For this review, take the finished solid that the model builds, in its own axes (mm). Face numbers are marked on the shaded views. A direction names the side the tool comes from. Give positions to 0.01 mm unless a question says otherwise; leave off trailing zeros. Write each loop counter-clockwise with the first axis right and the second up, starting at its lowest first coordinate (ties: lowest second). Pieces come first, ordered by that corner, then holes.
Q1. We need section D-D (z = -11.5). Write out the cut boundary in (x, y), then the cut area to 3 significant figures.
Q2. We need section B-B (z = 9). Write out the cut boundary in (x, y) (3 decimals), then the cut area to 3 significant figures.
Q3. Insertion check: P1, Ø6, axis at y = 54.5, z = 26, coming from the +X side; P2, Ø6.5, axis at x = 22.5, z = 34, coming from the +Y side; P3, Ø10, axis at y = 54, z = 25.5, coming from the -X side; P4, Ø12, axis at x = 4.5, z = 14.5, coming from the -Y side. Each pin has a flat end and moves straight along its axis. Give the tip position at first contact, or say it passes through.
Q4. Mouldability with a two-part tool opening along Y and no side actions: class the marked faces 1, 2 and 3 as released by +Y, released by -Y, zero draft, split by the parting line, or undercut.
Q5. We need section C-C (y = 0). Write out the cut boundary in (x, z), then the cut area to 3 significant figures.
Q6. We need section A-A (x = 0). Write out the cut boundary in (y, z), then the cut area to 3 significant figures.
Q7. Machinability: for the marked faces 4, 5 and 6, which of the approach directions +Z, -Z, +X, -X, +Y, -Y give a long, thin tool a straight path to every point of the face, cutting with its end or side? Answer none if there is none.
Q8. For line 1 (Z direction, x = 11, y = 32.5); line 2 (Y direction, x = 0, z = 17); line 3 (Z direction, x = 0, y = -19), list the stretches that pass through material, from the lowest coordinate up.
```python
from build123d import *

# Parameters (mm, degrees)
SKETCH1_R           = 30
SKETCH1_R_2         = 17.5
BOSS_EXTRUDE1_DEPTH = 38
BOSS_EXTRUDE2_START = -33
BOSS_EXTRUDE2_DEPTH = 33
SKETCH6_W           = 11
SKETCH6_H           = 36.919601085
BOSS_EXTRUDE3_DEPTH = 41.84
SKETCH8_R           = 5.835
CUT_EXTRUDE2_DEPTH  = 41.84
BOSS_EXTRUDE4_DEPTH = 11
SKETCH13_W          = 14
SKETCH13_H          = 10
BOSS_EXTRUDE7_DEPTH = 55
SKETCH14_W          = 5
SKETCH14_H          = 14
CUT_EXTRUDE3_DEPTH  = 2
BOSS_EXTRUDE8_DEPTH = 10
CUT_EXTRUDE4_DEPTH  = 100.425509369
SKETCH18_W          = 27.083405909
SKETCH18_H          = 15
CUT_EXTRUDE5_DEPTH  = 6


with BuildPart() as part:
    # Sketch1 → Boss-Extrude1 (new body)
    with BuildSketch(Plane.XY):
        Circle(SKETCH1_R)
        Circle(SKETCH1_R_2, mode=Mode.SUBTRACT)
    extrude(amount=BOSS_EXTRUDE1_DEPTH)

    # Sketch3 → Boss-Extrude2 (add)
    with BuildSketch(Plane.XY.offset(38).offset(BOSS_EXTRUDE2_START)):
        with BuildLine():
            Line((5, 29.580398915), (5, 66.5))
            Line((5, 66.5), (-5, 66.5))
            Line((-5, 66.5), (-5, 29.580398915))
            ThreePointArc((-5, 29.580398915), (0, 30), (5, 29.580398915))
        make_face()
    extrude(amount=BOSS_EXTRUDE2_DEPTH)

    # Sketch6 → Boss-Extrude3 (add)
    with BuildSketch(Plane(origin=(5, 0, 0), x_dir=(0, 0, -1), z_dir=(1, 0, 0))):
        with Locations((-10.5, 48.040199458)):
            Rectangle(SKETCH6_W, SKETCH6_H)
    extrude(amount=BOSS_EXTRUDE3_DEPTH)

    # Sketch8 → Cut-Extrude2 (cut)
    with BuildSketch(Plane.XY.offset(16)):
        with BuildLine():
            Line((38.535426242, 49.92600948), (19.843134833, 28.5))
            Line((19.843134833, 28.5), (19.843134833, 22.5))
            Line((19.843134833, 22.5), (50.730835644, 21.613123559))
            Line((50.730835644, 21.613123559), (58.316291642, 73.170252493))
            Line((58.316291642, 73.170252493), (32.080152152, 77.030302224))
            Line((32.080152152, 77.030302224), (31, 66.5))
            ThreePointArc((31, 66.5), (40.103293503, 60.638846144), (38.535426242, 49.92600948))
        make_face()
        with Locations((31, 56.5)):
            Circle(SKETCH8_R)
    extrude(amount=-CUT_EXTRUDE2_DEPTH, mode=Mode.SUBTRACT)

    # Sketch11 → Boss-Extrude4 (add)
    with BuildSketch(Plane(origin=(0, 0, 5), x_dir=(-1, 0, 0), z_dir=(0, 0, -1))):
        with BuildLine():
            Line((-19.843134833, 22.5), (-19.843134833, 28.5))
            Line((-19.843134833, 28.5), (-20.785686986, 29.580398915))
            Line((-20.785686986, 29.580398915), (-5, 29.580398915))
            ThreePointArc((-5, 29.580398915), (-12.91620491, 27.077142588), (-19.843134833, 22.5))
        make_face()
    extrude(amount=-BOSS_EXTRUDE4_DEPTH)

    # Sketch13 → Boss-Extrude7 (add)
    with BuildSketch(Plane.ZY.offset(5)):
        with Locations((12, 34.580398915)):
            Rectangle(SKETCH13_W, SKETCH13_H)
    extrude(amount=BOSS_EXTRUDE7_DEPTH)

    # Sketch14 → Cut-Extrude3 (cut)
    with BuildSketch(Plane(origin=(0, 39.580398915, 0), x_dir=(1, 0, 0), z_dir=(0, 1, 0))):
        with Locations((-7.5, -12)):
            Rectangle(SKETCH14_W, SKETCH14_H)
    extrude(amount=-CUT_EXTRUDE3_DEPTH, mode=Mode.SUBTRACT)

    # Sketch15 → Boss-Extrude8 (add)
    with BuildSketch(Plane(origin=(0, 39.580398915, 0), x_dir=(1, 0, 0), z_dir=(0, 1, 0))):
        with BuildLine():
            Line((-60, 10), (-60, -5))
            Line((-60, -5), (-32, -5))
            Line((-32, -5), (-32, 10))
            ThreePointArc((-32, 10), (-33.757359313, 14.242640687), (-38, 16))
            Line((-38, 16), (-42, 16))
            Line((-42, 16), (-42, 1))
            ThreePointArc((-42, 1), (-46, -3), (-50, 1))
            Line((-50, 1), (-50, 16))
            Line((-50, 16), (-54, 16))
            ThreePointArc((-54, 16), (-58.242640687, 14.242640687), (-60, 10))
        make_face()
    extrude(amount=-BOSS_EXTRUDE8_DEPTH)

    # Sketch16 → Cut-Extrude4 (cut, through all)
    with BuildSketch(Plane(origin=(0, 39.580398915, 0), x_dir=(1, 0, 0), z_dir=(0, 1, 0))):
        with BuildLine():
            ThreePointArc((-54, -19), (-58.242640687, -17.242640687), (-60, -13))
            Line((-60, -13), (-60, -19))
            Line((-60, -19), (-54, -19))
        make_face()
    extrude(amount=-CUT_EXTRUDE4_DEPTH, mode=Mode.SUBTRACT)

    # Sketch18 → Cut-Extrude5 (cut)
    with BuildSketch(Plane(origin=(0, 0, 0), x_dir=(-1, 0, 0), z_dir=(0, 0, -1))):
        with Locations((-23.74070021, 0)):
            Rectangle(SKETCH18_W, SKETCH18_H)
        with Locations((23.74070021, 0)):
            Rectangle(SKETCH18_W, SKETCH18_H)
    cut_extrude5 = extrude(amount=-CUT_EXTRUDE5_DEPTH, mode=Mode.SUBTRACT)

    # Mirror1: Cut-Extrude5 across plane
    add(cut_extrude5.mirror(Plane.XY.offset(19)), mode=Mode.SUBTRACT)


solid = part.part
```
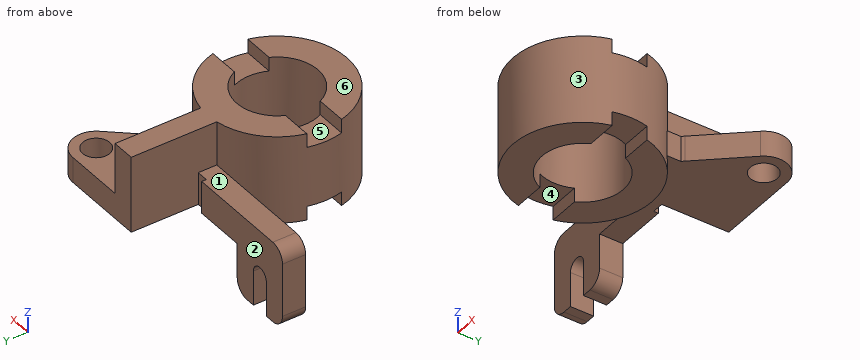
Computed:
1. outline: (-59.81, 29.58) - (-50, 29.58) - (-50, 39.58) - (-59.81, 39.58) - close; (-42, 29.58) - (-32.19, 29.58) - (-32.19, 39.58) - (-42, 39.58) - close
1. area: 196 mm2
2. outline: (-60, 29.58) - (-5, 29.58) arc R30 ccw (long way) to (19.843, 22.5) - (19.843, 28.5) - (38.535, 49.926) arc R10 ccw to (31, 66.5) - (-5, 66.5) - (-5, 37.58) - (-10, 37.58) - (-10, 39.58) - (-60, 39.58) - close; hole circle Ø35 at (0, 0); hole circle Ø11.67 at (31, 56.5)
2. area: 3,780 mm2
3. P1: stops at x = 5
3. P2: stops at y = 23.01
3. P3: stops at x = -5
3. P4: stops at y = -30
4. face 1: zero draft
4. face 2: released by +Y
4. face 3: undercut
5. outline: (-30, 6) - (-17.5, 6) - (-17.5, 32) - (-30, 32) - close; (17.5, 6) - (30, 6) - (30, 32) - (17.5, 32) - close
5. area: 650 mm2
6. outline: (-30, 0) - (-17.5, 0) - (-17.5, 38) - (-30, 38) - close; (17.5, 0) - (30, 0) - (30, 5) - (66.5, 5) - (66.5, 38) - (17.5, 38) - close
6. area: 2,150 mm2
7. face 4: -Z, +X, -X
7. face 5: +Z, +X, -X
7. face 6: +Z, +X, -X, +Y, -Y
8. line 1: z = 5 to 16
8. line 2: y = -30 to -17.5, 17.5 to 66.5
8. line 3: z = 0 to 38
